Geometry: final body of the model. Coordinates: model frame, mm. Face numbers are marked on the shaded views. A direction names the side the tool comes from. Give positions to 0.01 mm unless a question says otherwise; leave off trailing zeros. Write each loop counter-clockwise with the first axis right and the second up, starting at its lowest first coordinate (ties: lowest second). Pieces come first, ordered by that corner, then holes. Notation, with made-up numbers: (-7.5, 4) -> (43.5, 4) arc R15 ccw to (43.5, 27) -> close; hole circle Ø11 at (-36.75, -33). An arc over 180 degrees is marked (long way). Use CSV: the item, a comma, the result in double quotes. Start each with the question number.
1) Section B-B (z = 0). Output: boundary loops of the cut face in (x, y), plus the area to 3 significant figures.
2) Set-up query: the marked faces 1 and 2. Return all of +Z, -Z, +X, -X, +Y, -Y with unobstructed straight access to the full face (end or side cutting, diameter ignored); none if empty.
3) Section A-A (x = 0). Output: boundary loops of the cut face in (y, z), plus the area to 3 significant figures.
4) Material intervals for line 1 (Z direction, x = 0, y = 1.25); line 2 (Z direction, x = 0, y = -3.5); line 3 (X direction, y = -6.75, z = 17), sorted ascending. Write a range as [from, to].
5) Contact query for flat-ended pins moving along their axis: P1, Ø6, axis at x = -34, y = 1, coming from the +Z side; P2, Ø5, axis at x = 0, z = 33, coming from the -Y side; P3, Ø3, axis at y = 1, z = 57, coming from the +X side; P4, Ø1, axis at x = -11, y = -3, coming from the +Z side. Output: stop coordinate, or through.
6) Section C-C (z = 33). Output: boundary loops of the cut face in (x, y), plus the area to 3 significant figures.
7) Section D-D (y = -3.25). Count the separate pieces of the cut face and the enclosed holes in it, plus the area to 3 significant figures.
```python
from build123d import *

# Parameters (mm, degrees)
F0_R            = 82
F0_R_2          = 56
F0_R_3          = 6
F0_R_4          = 27.5
F0_R_5          = 3
F1_DEPTH        = 8
F2_DEPTH        = 4
F3_DEPTH        = 8
F3_COPIES_COUNT = 5
F4_R            = 3
F5_DEPTH        = 12
F5_COPIES_COUNT = 4


# Not quite as in the source:
# - a pattern or mirror of a feature is missing from the dataset's text; its kind, count and spacing are read off the source's solid


with BuildPart() as f1:
    # F0 (on Front) → F1 (new body)
    with BuildSketch(Plane.XZ):
        Circle(F0_R)
        Circle(F0_R_2, mode=Mode.SUBTRACT)
        with Locations((0, 69)):
            Circle(F0_R_3, mode=Mode.SUBTRACT)
        Circle(F0_R_2)
        Circle(F0_R_4, mode=Mode.SUBTRACT)
        with Locations((0, 33)):
            Circle(F0_R_5, mode=Mode.SUBTRACT)
        with Locations((0, 69)):
            Circle(F0_R_3)
        with Locations((0, 33)):
            Circle(F0_R_5)
    extrude(amount=F1_DEPTH)

    # F0 (on Front) → F2 (join)
    with BuildSketch(Plane.XZ):
        Circle(F0_R_2)
        Circle(F0_R_4, mode=Mode.SUBTRACT)
        with Locations((0, 33)):
            Circle(F0_R_5, mode=Mode.SUBTRACT)
        with Locations((0, 33)):
            Circle(F0_R_5)
    extrude(amount=-F2_DEPTH)

    # F0 (on Front) → F3 (cut)
    with BuildSketch(Plane.XZ):
        with Locations((0, 69)):
            Circle(F0_R_3)
    f3 = extrude(amount=F3_DEPTH, mode=Mode.SUBTRACT)

    # F3_copies: F3 ×5 about axis
    f3_copies_axis = Axis((0, 0, 0), (0, 1, 0))
    for i in range(1, F3_COPIES_COUNT):
        add(f3.rotate(f3_copies_axis, i * 360 / F3_COPIES_COUNT), mode=Mode.SUBTRACT)

    # F4 (on face) → F5 (cut)
    with BuildSketch(Plane(origin=(0, 4, 0), x_dir=(-1, 0, 0), z_dir=(0, 1, 0))):
        with Locations((0, 33)):
            Circle(F4_R)
    f5 = extrude(amount=-F5_DEPTH, mode=Mode.SUBTRACT)

    # F5_copies: F5 ×4 about axis
    f5_copies_axis = Axis((0, 0, 0), (0, 1, 0))
    for i in range(1, F5_COPIES_COUNT):
        add(f5.rotate(f5_copies_axis, i * 360 / F5_COPIES_COUNT), mode=Mode.SUBTRACT)


solid = f1.part
```
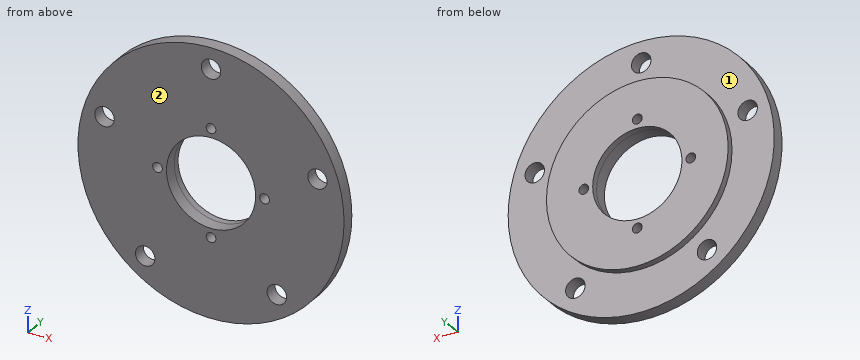
Answers follow:
1,outline,"(-82, -8) -> (-36, -8) -> (-36, 4) -> (-56, 4) -> (-56, 0) -> (-82, 0) -> close; (-30, -8) -> (-27.5, -8) -> (-27.5, 4) -> (-30, 4) -> close; (27.5, -8) -> (30, -8) -> (30, 4) -> (27.5, 4) -> close; (36, -8) -> (82, -8) -> (82, 0) -> (56, 0) -> (56, 4) -> (36, 4) -> close"
1,area,"956 mm^2"
2,face 1,"+Y"
2,face 2,"+Z, -Z, +X, -X, -Y"
3,outline,"(-8, -82) -> (0, -82) -> (0, -56) -> (4, -56) -> (4, -36) -> (-8, -36) -> close; (-8, -30) -> (4, -30) -> (4, -27.5) -> (-8, -27.5) -> close; (-8, 27.5) -> (4, 27.5) -> (4, 30) -> (-8, 30) -> close; (-8, 36) -> (4, 36) -> (4, 56) -> (0, 56) -> (0, 63) -> (-8, 63) -> close; (-8, 75) -> (0, 75) -> (0, 82) -> (-8, 82) -> close"
3,area,"860 mm^2"
4,line 1,"z = [-56, -36], [-30, -27.5], [27.5, 30], [36, 56]"
4,line 2,"z = [-82, -36], [-30, -27.5], [27.5, 30], [36, 63], [75, 82]"
4,line 3,"x = [-80.22, -69.78], [-61.46, -21.62], [21.62, 61.46], [69.78, 80.22]"
5,P1,"stops at z = 75.84"
5,P2,"passes through"
5,P3,"stops at x = 60.01"
5,P4,"stops at z = 81.32"
6,outline,"(-75.07, -8) -> (-3, -8) -> (-3, 4) -> (-45.24, 4) -> (-45.24, 0) -> (-75.07, 0) -> close; (3, -8) -> (75.07, -8) -> (75.07, 0) -> (45.24, 0) -> (45.24, 4) -> (3, 4) -> close"
6,area,"1,490 mm^2"
7,separate pieces,"1"
7,enclosed holes,"10"
7,area,"18,100 mm^2"
